For this review, use the dimensioned drawing (mm, ordinates from the lowest corner) and the shaded views. A direction names the side the tool comes from. Coordinates: 2 decimals unless noted, no trailing zeros. Order: outer loops, then holes, each group sorted by start corner. A loop starts at its lowest first (then second) coordinate and runs counter-clockwise, first axis right, second up. Notation, with made-up numbers: (87, 50) -> (123, 50) arc R23 ccw to (123, 81) -> close; hole circle Ø11 at (15.5, -5.5). An arc over 180 degrees is marked (long way). Return JSON: item names as keys, results as strings. Group by question number.
Item 1: Insertion check: pin 1 (2 mm diameter, centred on y = 20, z = 7, fed in from -X); pin 2 (1.5 mm diameter, centred on y = 3, z = 6, fed in from -X); pin 3 (2 mm diameter, centred on y = 16.5, z = 1.5, fed in from -X). Each pin has a flat end and moves straight along its axis. Give the tip position at first contact, or say it passes through.
Item 2: For line 1 along Y through (x, z) = (4.75, 5); line 2 along Z through (x, y) = (4.75, 17); line 3 along Z through (x, y) = (5, 4.5), list the stretches that pass through material, from the lowest coordinate up.
Item 3: Draft analysis for pull direction X (two halves, no side actions). For the marked faces 5, 6 and 7, state which applies: +X half, -X half, draft (parallel to the pull), parting line (faces both ways), or undercut.
Item 4: Machinability: for the marked faces 1, 2, 3 and 4, which of the approach directions +Z, -Z, +X, -X, +Y, -Y give a long, thin tool a straight path to every point of the face, cutting with its end or side? Answer none if there is none.
Item 5: Take a section at B-B (y = 17). Write out the cut boundary in (x, z).
Item 6: Take a section at C-C (y = 9.75). Write out the cut boundary in (x, z).
Item 7: Take a section at A-A (y = 3.25). Write out the cut boundary in (x, z).
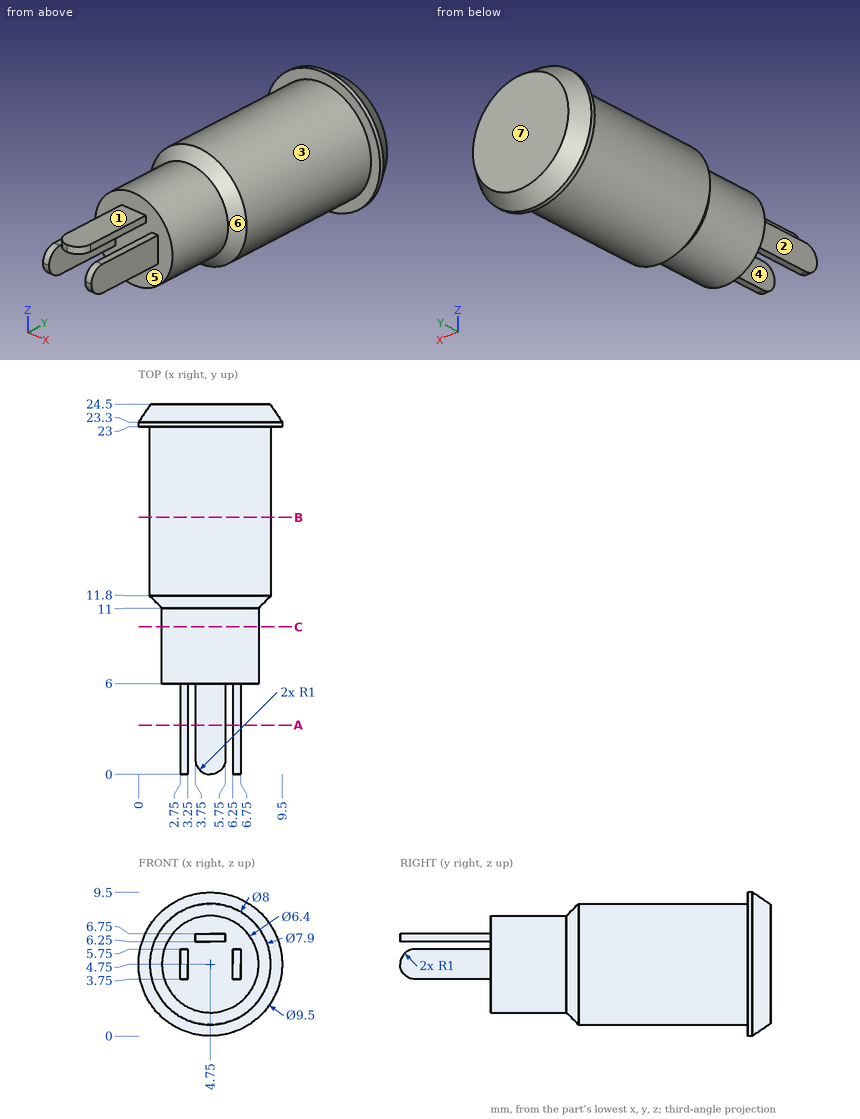
Findings below:
{
 "1": {"pin 1": "stops at x = 0.95", "pin 2": "stops at x = 2.75", "pin 3": "stops at x = 1.44"},
 "2": {"line 1": "y = 6 to 24.5", "line 2": "z = 0.75 to 8.75", "line 3": "z = 6.25 to 6.75"},
 "3": {"face 5": "undercut", "face 6": "parting line", "face 7": "draft"},
 "4": {"face 1": "+Z, +X, -X, -Y", "face 2": "+Z, -Z, -X, -Y", "face 3": "-Y", "face 4": "+Z, -Z, -Y"},
 "5": {"outline": "circle Ø8 at (4.75, 4.75)"},
 "6": {"outline": "circle Ø6.4 at (4.75, 4.75)"},
 "7": {"outline": "(2.75, 3.75) -> (3.25, 3.75) -> (3.25, 5.75) -> (2.75, 5.75) -> close; (3.75, 6.25) -> (5.75, 6.25) -> (5.75, 6.75) -> (3.75, 6.75) -> close; (6.25, 3.75) -> (6.75, 3.75) -> (6.75, 5.75) -> (6.25, 5.75) -> close"}
}
